from build123d import *

# Parameters (mm, degrees)
DODANIE_WYCI_GNI_CIE1_DEPTH = 12.3
ZAOKR_GLENIE1_R             = 0.2
ZAOKR_GLENIE2_R             = 1
DODANIE_WYCI_GNI_CIE2_DEPTH = 4.4
SZKIC3_R                    = 2.45
WYTNIJ_WYCI_GNI_CIE1_DEPTH  = 3.2
WYTNIJ_WYCI_GNI_CIE2_REACH  = 38.556


with BuildPart() as part:
    # Szkic1 → Dodanie-wyciągnięcie1 (new body)
    with BuildSketch(Plane(origin=(0, 0, 0), x_dir=(0, 0, -1), z_dir=(1, 0, 0))):
        Polygon((0, 0), (0, 23.4), (16.2, 23.4), (16.2, 28.3), (19.6, 28.3), (19.6, 23.4), (23.7, 23.4), (23.7, 0), (19.6, 0), (19.6, -4.9), (16.2, -4.9), (16.2, 0), align=None)
    extrude(amount=DODANIE_WYCI_GNI_CIE1_DEPTH)

    # Zaokrąglenie1
    zaokr_glenie1_edges = [part.edges().sort_by_distance(p)[0] for p in [
        (0, 11.7, 0),
        (0, 23.4, -8.1),
        (0, 25.85, -19.6),
        (0, 23.4, -21.65),
        (0, 11.7, -23.7),
        (0, 0, -21.65),
        (0, -2.45, -19.6),
        (0, 0, -8.1),
        (12.3, -2.45, -19.6),
        (6.15, 0, 0),
        (6.15, 23.4, 0),
        (12.3, 0, -21.65),
        (6.15, 28.3, -19.6),
        (6.15, 23.4, -23.7),
        (6.15, 0, -23.7),
        (6.15, -4.9, -19.6),
        (12.3, 11.7, -23.7),
        (12.3, 23.4, -21.65),
        (12.3, 25.85, -19.6),
        (12.3, 23.4, -8.1),
        (12.3, 11.7, 0),
        (12.3, 0, -8.1),
    ]]
    fillet(zaokr_glenie1_edges, radius=ZAOKR_GLENIE1_R)

    # Zaokrąglenie2
    # the kernel refuses this fillet: 1 mm, written as the material it takes off along each edge
    with BuildSketch(Plane(origin=(11.3, 27.3, -19.6), x_dir=(0, 1, 0), z_dir=(-1, 0, 0))) as zaokr_glenie2_piece_1:
        with BuildLine():
            CenterArc((0.8, -0.2), 0.2, 0, 90)
            Line((1, -0.2), (1, 0))
            Line((1, 0), (0.8, 0))
        make_face()
    revolve(axis=Axis((11.3, 27.3, -19.6), (0, 0, -1)), revolution_arc=90, mode=Mode.SUBTRACT)
    with BuildSketch(Plane(origin=(1, 27.3, -19.6), x_dir=(-1, 0, 0), z_dir=(0, -1, 0))) as zaokr_glenie2_piece_2:
        with BuildLine():
            CenterArc((0.8, -0.2), 0.2, 0, 90)
            Line((1, -0.2), (1, 0))
            Line((1, 0), (0.8, 0))
        make_face()
    revolve(axis=Axis((1, 27.3, -19.6), (0, 0, -1)), revolution_arc=90, mode=Mode.SUBTRACT)
    with BuildSketch(Plane(origin=(11.3, -3.9, -19.6), x_dir=(1, 0, 0), z_dir=(0, 1, 0))) as zaokr_glenie2_piece_3:
        with BuildLine():
            CenterArc((0.8, -0.2), 0.2, 0, 90)
            Line((1, -0.2), (1, 0))
            Line((1, 0), (0.8, 0))
        make_face()
    revolve(axis=Axis((11.3, -3.9, -19.6), (0, 0, -1)), revolution_arc=90, mode=Mode.SUBTRACT)
    with BuildSketch(Plane(origin=(1, -3.9, -19.6), x_dir=(0, -1, 0), z_dir=(1, 0, 0))) as zaokr_glenie2_piece_4:
        with BuildLine():
            CenterArc((0.8, -0.2), 0.2, 0, 90)
            Line((1, -0.2), (1, 0))
            Line((1, 0), (0.8, 0))
        make_face()
    revolve(axis=Axis((1, -3.9, -19.6), (0, 0, -1)), revolution_arc=90, mode=Mode.SUBTRACT)
    with BuildSketch(Plane(origin=(12.3, -4.9, -19.6), x_dir=(-1, 0, 0), z_dir=(0, 0, 1)), Plane(origin=(0, -4.9, -19.6), x_dir=(0, 1, 0), z_dir=(0, 0, 1)), Plane(origin=(0, 28.3, -13.7), x_dir=(0, -1, 0), z_dir=(0, 0, -1)), Plane(origin=(12.3, 28.3, -13.7), x_dir=(-1, 0, 0), z_dir=(0, 0, -1))) as zaokr_glenie2_piece_5:
        with BuildLine():
            CenterArc((ZAOKR_GLENIE2_R, -ZAOKR_GLENIE2_R), ZAOKR_GLENIE2_R, 90, 90)
            Line((0, -ZAOKR_GLENIE2_R), (0, 0))
            Line((0, 0), (ZAOKR_GLENIE2_R, 0))
        make_face()
    extrude(amount=5.9, mode=Mode.SUBTRACT)

    # Szkic2 → Dodanie-wyciągnięcie2 (add)
    with BuildSketch(Plane(origin=(0, 0, -23.7), x_dir=(-1, 0, 0), z_dir=(0, 0, -1))):
        with BuildLine():
            Line((-3.65, 13.1), (-3.65, 11.128078794))
            ThreePointArc((-3.65, 11.128078794), (-6.15, 0.2), (-8.65, 11.128078794))
            Line((-8.65, 11.128078794), (-8.65, 13.1))
            ThreePointArc((-8.65, 13.1), (-6.15, 15.6), (-3.65, 13.1))
        make_face()
    extrude(amount=DODANIE_WYCI_GNI_CIE2_DEPTH)

    # Szkic3 → Wytnij-wyciągnięcie1 (cut)
    with BuildSketch(Plane(origin=(0, 0, -28.1), x_dir=(-1, 0, 0), z_dir=(0, 0, -1))):
        with Locations((-6.15, 5.95)):
            Circle(SZKIC3_R)
    extrude(amount=-WYTNIJ_WYCI_GNI_CIE1_DEPTH, mode=Mode.SUBTRACT)

    # Szkic5 → Wytnij-wyciągnięcie2 (cut, up to next)
    with BuildSketch(Plane(origin=(0, 0, -19.6), x_dir=(-1, 0, 0), z_dir=(0, 0, -1)), mode=Mode.PRIVATE) as wytnij_wyci_gni_cie2_sk1:
        with BuildLine():
            Line((-5.5, 26.759934208), (-5.5, 28.3))
            Line((-5.5, 28.3), (-6.8, 28.3))
            Line((-6.8, 28.3), (-6.8, 26.759934208))
            ThreePointArc((-6.8, 26.759934208), (-6.15, 25), (-5.5, 26.759934208))
        make_face()
    wytnij_wyci_gni_cie2_tool1 = extrude(wytnij_wyci_gni_cie2_sk1.sketch, amount=-WYTNIJ_WYCI_GNI_CIE2_REACH, mode=Mode.PRIVATE) & part.part
    wytnij_wyci_gni_cie2 = wytnij_wyci_gni_cie2_tool1.solids().sort_by_distance((6.15, 26.584181, -19.6))[0]
    add(wytnij_wyci_gni_cie2, mode=Mode.SUBTRACT)

    # Lustro1: Wytnij-wyciągnięcie2 across plane
    add(wytnij_wyci_gni_cie2.mirror(Plane.ZX.offset(11.7)), mode=Mode.SUBTRACT)


solid = part.part
The listing builds one solid part. Answer for the finished solid, in the listing's coordinates (mm). A direction names the side the tool comes from. Coordinates: 2 decimals unless noted, no trailing zeros. Write each loop counter-clockwise with the first axis right and the second up, starting at its lowest first coordinate (ties: lowest second). Pieces come first, ordered by that corner, then holes. Notation, with made-up numbers: (84, 52.25) - (135, 52.25) arc R14 ccw to (135, 59.25) - close; hole circle Ø9 at (14.5, 43.5). An arc over 180 degrees is marked (long way). Put each result on its own line as item: value.
1. The part is cut by section C-C on y = 20. Give the vertices of the cut face in (x, z).
Answer sheet:
outline: (0, -23.5) arc R0.2 ccw to (0.2, -23.7) - (12.1, -23.7) arc R0.2 ccw to (12.3, -23.5) - (12.3, -0.2) arc R0.2 ccw to (12.1, 0) - (0.2, 0) arc R0.2 ccw to (0, -0.2) - close
2. The part is cut by section B-B on z = -20.75. Give the vertices of the cut face in (x, y).
Answer sheet:
outline: (0, 0.2) arc R0.2 ccw to (0.2, 0) - (12.1, 0) arc R0.2 ccw to (12.3, 0.2) - (12.3, 23.2) arc R0.2 ccw to (12.1, 23.4) - (0.2, 23.4) arc R0.2 ccw to (0, 23.2) - close
3. The part is cut by section A-A on y = 26. Give the vertices of the cut face in (x, z), plus the area to 3 significant figures.
Answer sheet:
outline: (0, -19.4) arc R0.2 ccw to (0.2, -19.6) - (5.15, -19.6) - (5.15, -16.2) - (0, -16.2) - close; (7.15, -19.6) - (12.1, -19.6) arc R0.2 ccw to (12.3, -19.4) - (12.3, -16.2) - (7.15, -16.2) - close
area: 35.0 mm^2
4. Find the intervals of material crossed by line 1 along X through (y, z) = (-2.6, -17.9); line 2 along Y through (x, z) = (6.15, -26.6); line 3 along Y through (x, z) = (6.15, -18.55), in increasing order. Write a range as from..to.
Answer sheet:
line 1: x = 0..5.15, 7.15..12.3
line 2: y = 0.2..3.5, 8.4..15.6
line 3: y = -1.6..25
5. A tool of negligible diameter and unlimited length cuts with its end or side. For faces 1 (the face through (6, 23.4, -22)), 2 (the face through (6.2, 25, -17.9)), 3 (the face through (0.285, -4.599, -17.822)), 4 (the face through (8.65, 12, -26)), 5 (the face through (6.8, -4, -18)), from which of +Z, -Z, +X, -X, +Y, -Y can it reach the whole face along a straight path? Write none if from no direction.
Answer sheet:
face 1: -Z, +X, -X, +Y
face 2: +Z, -Z
face 3: +Z, -Z, -X, -Y
face 4: -Z, +X, +Y
face 5: +Z, -Z, -Y
6. The part is cut by section D-D on x = 9.5. Give the vertices of the cut face in (y, z).
Answer sheet:
outline: (-4.9, -19.4) arc R0.2 ccw to (-4.7, -19.6) - (0, -19.6) - (0, -23.5) arc R0.2 ccw to (0.2, -23.7) - (1.28, -23.7) - (1.28, -28.1) - (10.62, -28.1) - (10.62, -23.7) - (23.2, -23.7) arc R0.2 ccw to (23.4, -23.5) - (23.4, -19.6) - (28.1, -19.6) arc R0.2 ccw to (28.3, -19.4) - (28.3, -16.2) - (23.4, -16.2) - (23.4, -0.2) arc R0.2 ccw to (23.2, 0) - (0.2, 0) arc R0.2 ccw to (0, -0.2) - (0, -16.2) - (-4.9, -16.2) - close
7. Determine the mould class of faces 6 (the face through (5.933, 0.204, -25.869)), 7 (the face through (6, 17, -23.7)), 8 (the face through (6.8, 28, -18)) for opening direction X: pulls with the +X half, pulls with the -X half, needs draft (parallel to the pull), parting line crosses it, or undercut.
Answer sheet:
face 6: parting line crosses it
face 7: needs draft
face 8: undercut
8. Flat-ended cylindrical pins translate along their axes: pin 1 Ø1.6 at (y, z) = (12, -25.5) entering from +X; pin 2 Ø4.5 at (x, z) = (9, -21.5) entering from -Y; pin 3 Ø1.5 at (x, y) = (3.5, -0.5) entering from -Z; pin 4 Ø0.5 at (y, z) = (28, -17.5) entering from -X. Find the tip coordinate at first contact, or state that the pin passes through.
Answer sheet:
pin 1: stops at x = 8.65
pin 2: stops at y = -4.9
pin 3: stops at z = -23.7
pin 4: stops at x = 0.11
